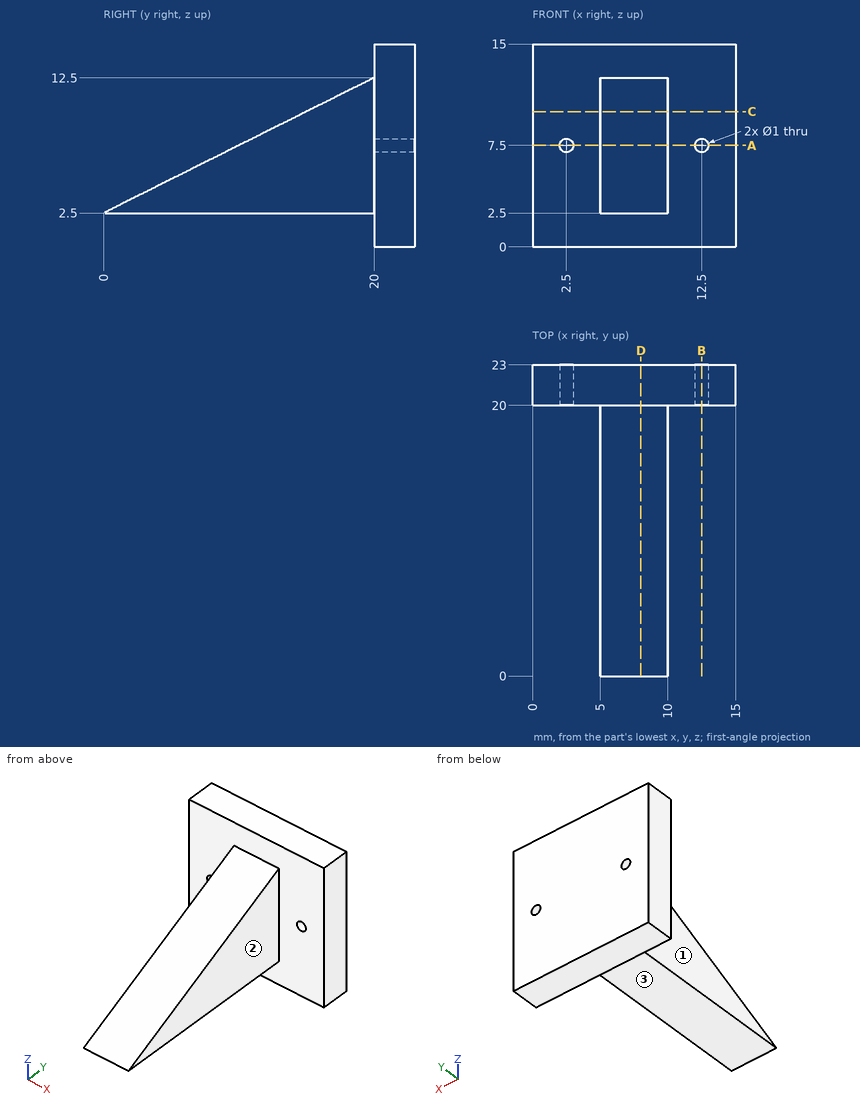
The figure shows three views and two pictorial views of one solid part (mm, origin at its lowest corner). Answer the questions. A direction names the side the tool comes from. Coordinates: 2 decimals unless noted, no trailing zeros. Loops run counter-clockwise (first coordinate to the right, second up) from the corner with the lowest first, then second, coordinate; pieces in that order, holes last. Notation, with made-up numbers: (58, -7.75) -> (78, -7.75) arc R21 ccw to (78, 27.25) -> close; hole circle Ø9 at (-4.75, 5). An arc over 180 degrees is marked (long way). Return JSON: item names as keys, results as strings. Group by question number.
(1) Find the intervals of material crossed by probe 1 along X at (y, z) = (21.95, 7.5); probe 2 along Y at (x, z) = (1.75, 12.5); probe 3 along X at (y, z) = (12, 6), in increasing order. Write a range as from..to.
(2) A cutting plane is placed at B-B on x = 12.5. Write down the section's boundary in (y, z), and give its area (3 significant figures).
(3) A cutting plane is placed at C-C on z = 10. Write down the section's boundary in (x, y), and give its area (3 significant figures).
(4) Given pin 1 Ø4 at (x, y) = (7.5, 13.5) entering from -Z; pin 2 Ø1 at (x, z) = (11.5, 3) entering from -Y; pin 3 Ø5 at (x, y) = (4.5, 9.5) entering from +Z, each flat-ended and moving along its own axis, determine where each tip first touches the part or whether it passes through.
(5) A cutting plane is placed at D-D on x = 8. Write down the section's boundary in (y, z), and give its area (3 significant figures).
(6) A cutting plane is placed at A-A on z = 7.5. Write down the section's boundary in (x, y), and give its area (3 significant figures).
(7) Which of the six approach directions +Z, -Z, +X, -X, +Y, -Y give full straight-line access (tool end or side, diameter ignored) to the marked faces 1, 2 and 3?
The answers:
{
 "1": {"probe 1": "x = 0..2, 3..12, 13..15", "probe 2": "y = 20..23", "probe 3": "x = 5..10"},
 "2": {"outline": "(20, 0) -> (23, 0) -> (23, 7) -> (20, 7) -> close; (20, 8) -> (23, 8) -> (23, 15) -> (20, 15) -> close", "area": "42.0 mm^2"},
 "3": {"outline": "(0, 20) -> (5, 20) -> (5, 15) -> (10, 15) -> (10, 20) -> (15, 20) -> (15, 23) -> (0, 23) -> close", "area": "70.0 mm^2"},
 "4": {"pin 1": "stops at z = 2.5", "pin 2": "stops at y = 20", "pin 3": "stops at z = 8.47"},
 "5": {"outline": "(0, 2.5) -> (20, 2.5) -> (20, 0) -> (23, 0) -> (23, 15) -> (20, 15) -> (20, 12.5) -> close", "area": "145 mm^2"},
 "6": {"outline": "(0, 20) -> (2, 20) -> (2, 23) -> (0, 23) -> close; (3, 20) -> (5, 20) -> (5, 10) -> (10, 10) -> (10, 20) -> (12, 20) -> (12, 23) -> (3, 23) -> close; (13, 20) -> (15, 20) -> (15, 23) -> (13, 23) -> close", "area": "89.0 mm^2"},
 "7": {"face 1": "+Z, -Z, -X, -Y", "face 2": "+Z, -Z, +X, -Y", "face 3": "-Z, +X, -X, -Y"}
}
